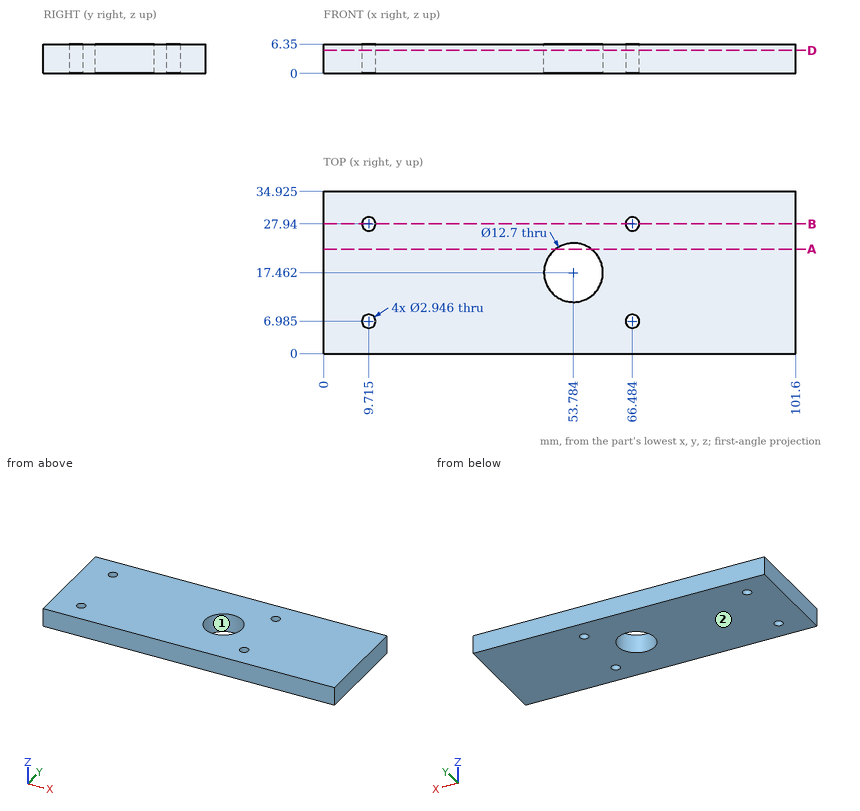
Verification items for this drawing (mm, ordinates from the low corner). Give positions to 0.01 mm unless a question says otherwise; leave off trailing zeros. Write each loop counter-clockwise with the first axis right and the second up, starting at its lowest first coordinate (ties: lowest second). Pieces come first, ordered by that corner, then holes.
1) Release check for a two-part mould opening along X. For the marked faces 1 and 2 record: pulls with the +X half, pulls with the -X half, needs draft (parallel to the pull), parting line crosses it, or undercut.
2) Material ranges on L1, parallel to X at y = 27, z = 3.5; L2, parallel to X at y = 29, z = 1 (1 decimal); L3, parallel to Y at x = 59, z = 3.75 (1 decimal), recorded low to high.
3) Section check D-D, the plane z = 5. State how many separate pieces and enclosed holes the cut face has, and give its area (3 significant figures).
4) Section check B-B, the plane y = 27.94. Record the boundary of the cut face in (x, z), and give its area (3 significant figures).
5) Section check A-A, the plane y = 22.5. Record the boundary of the cut face in (x, z), and give its area (3 significant figures).
Computed:
1. face 1: undercut
1. face 2: needs draft
2. L1: x = 0 to 8.58, 10.85 to 65.35, 67.62 to 101.6
2. L2: x = 0 to 8.7, 10.7 to 65.5, 67.5 to 101.6
2. L3: y = 0 to 13.8, 21.1 to 34.9
3. separate pieces: 1
3. enclosed holes: 5
3. area: 3,390 mm2
4. outline: (0, 0) - (8.24, 0) - (8.24, 6.35) - (0, 6.35) - close; (11.19, 0) - (65.01, 0) - (65.01, 6.35) - (11.19, 6.35) - close; (67.96, 0) - (101.6, 0) - (101.6, 6.35) - (67.96, 6.35) - close
4. area: 608 mm2
5. outline: (0, 0) - (49.92, 0) - (49.92, 6.35) - (0, 6.35) - close; (57.65, 0) - (101.6, 0) - (101.6, 6.35) - (57.65, 6.35) - close
5. area: 596 mm2
